Here's how the part is built. I have some questions about the finished solid (model axes, mm). Face numbers are marked on the shaded views. A direction names the side the tool comes from. Round coordinates to 2 decimals unless told otherwise and drop trailing zeros. Order: outer loops, then holes, each group sorted by start corner. A loop starts at its lowest first (then second) coordinate and runs counter-clockwise, first axis right, second up. Notation, with made-up numbers: (67, 8.5) -> (118, 8.5) arc R27 cw to (118, 27.5) -> close; hole circle Ø6 at (-19.5, 0). An arc over 180 degrees is marked (long way). Use a Markdown table: item, result. Add a question column.
(1) I want a section at C-C, the plane x = 30.5. Please give me the cut outline in (y, z), then the cut area to 3 significant figures.
(2) I'm going to push flat-ended pins straight in: P1, Ø3.5, axis at x = 8, z = -33.18, coming from the +Y side; P2, Ø1, axis at x = 62.5, z = -46.5, coming from the -Y side; P3, Ø2.5, axis at x = 26, z = 17.32, coming from the +Y side. Where does each tip first touch, or does it pass through?
(3) If I drill on probe 1 along Y at (x, z) = (73, -17); probe 2 along X at (y, z) = (8, -62); probe 3 along Z at (x, y) = (42, 6), over which ranges is the centre line in solid material (lowest first)?
(4) Thinking about a two-plate mould opening in Y: for the marked faces 1, 2 and 3, which applies, pulls with the +Y half, pulls with the -Y half, needs draft (parallel to the pull), parting line crosses it, or undercut?
(5) On a 3-axis mill with a long thin cutter (end or side, diameter ignored), from which of +Z, -Z, +X, -X, +Y, -Y can I reach the whole of each face in a straight line? I mean the marked faces 4, 5 and 6. Say none if no direction works.
(6) I want a section at D-D, the plane z = -47. Please give me the cut outline in (x, y), then the cut area to 3 significant figures.
(7) I want a section at B-B, the plane x = 40. Give the number of separate pieces and of enclosed holes in the cut face, then the cut area to 3 significant figures.
(8) I want a section at A-A, the plane z = 4. Please give me the cut outline in (x, y), then the cut area to 3 significant figures.
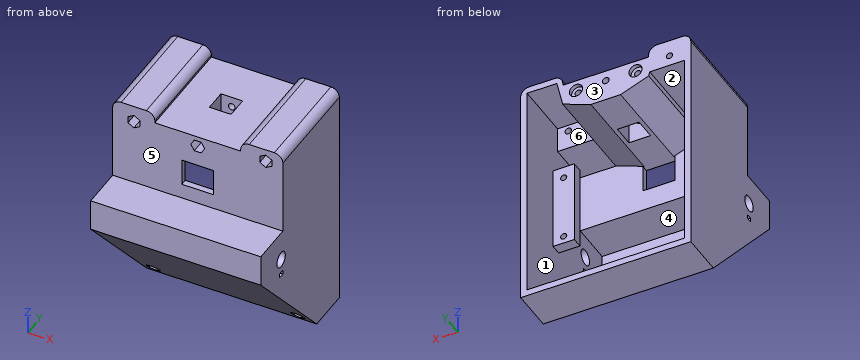
from build123d import *

# Parameters (mm, degrees)
BOSS_EXTRUDE1_DEPTH = 80
SHELL1_T            = -3
SKETCH3_W           = 46
SKETCH3_H           = 47
BOSS_EXTRUDE2_DEPTH = 17
SKETCH4_W           = 10.2
SKETCH4_H           = 10.2
CUT_EXTRUDE1_DEPTH  = 20
SKETCH6_W           = 15
SKETCH6_H           = 12.8
CUT_EXTRUDE2_DEPTH  = 3
SKETCH7_W           = 40.4
SKETCH7_H           = 50
CUT_EXTRUDE3_DEPTH  = 5
FILLET1_R           = 4
CUT_EXTRUDE7_DEPTH  = 47
SKETCH13_R          = 1.5
CUT_EXTRUDE8_DEPTH  = 25
SKETCH14_R          = 3.1
CUT_EXTRUDE9_DEPTH  = 2
SKETCH17_W          = 45
SKETCH17_H          = 5
BOSS_EXTRUDE5_DEPTH = 74
CUT_EXTRUDE10_REACH = 126.093
SKETCH18_W          = 54
SKETCH18_H          = 45
CUT_EXTRUDE11_REACH = 126.093
SKETCH19_R          = 1.45
BOSS_EXTRUDE6_DEPTH = 47
SKETCH22_R          = 1.45
CUT_EXTRUDE12_DEPTH = 135.415364765
SKETCH24_R          = 3.7
SKETCH24_W          = 2
SKETCH24_H          = 3
CUT_EXTRUDE13_DEPTH = 125.856940719
BOSS_EXTRUDE7_DEPTH = 74
SKETCH27_R          = 1.5
CUT_EXTRUDE14_DEPTH = 10
CUT_EXTRUDE15_START = -3
CUT_EXTRUDE15_DEPTH = 32
CUT_EXTRUDE16_DEPTH = 30
BOSS_EXTRUDE8_DEPTH = 20
SKETCH31_R          = 1.5
CUT_EXTRUDE17_DEPTH = 123.649786567
CUT_EXTRUDE18_DEPTH = 15
CUT_EXTRUDE19_REACH = 126.093
SKETCH33_W          = 10
SKETCH33_H          = 5
SKETCH34_R          = 1.6
CUT_EXTRUDE20_DEPTH = 135.415364765
CUT_EXTRUDE22_DEPTH = 14


with BuildPart() as part:
    # Sketch2 → Boss-Extrude1 (new body)
    with BuildSketch(Plane(origin=(0, 0, 0), x_dir=(0, 0, -1), z_dir=(1, 0, 0))):
        Polygon((-27.320490368, 20.998248687), (-27.320490368, -29.001751313), (12.679509632, -29.001751313), (12.679509632, -48.511383538), (27.679509632, -48.511383538), (82.679509632, 0.998248687), (82.679509632, 20.998248687), align=None)
    extrude(amount=BOSS_EXTRUDE1_DEPTH)

    # Shell1
    shell1_openings = [part.faces().sort_by_distance(p)[0] for p in [
        (40, 20.998248687, -27.679509632),
    ]]
    offset(amount=SHELL1_T, openings=shell1_openings, kind=Kind.INTERSECTION)

    # Sketch3 → Boss-Extrude2 (add)
    with BuildSketch(Plane(origin=(0, 0, 24.320490368), x_dir=(-1, 0, 0), z_dir=(0, 0, -1))):
        with Locations((-40, -2.501751313)):
            Rectangle(SKETCH3_W, SKETCH3_H)
    extrude(amount=BOSS_EXTRUDE2_DEPTH)

    # Sketch4 → Cut-Extrude1 (cut)
    with BuildSketch(Plane.XY.offset(27.320490368)):
        with Locations((40, -4.001751313)):
            Rectangle(SKETCH4_W, SKETCH4_H)
    extrude(amount=-CUT_EXTRUDE1_DEPTH, mode=Mode.SUBTRACT)

    # Sketch6 → Cut-Extrude2 (cut)
    with BuildSketch(Plane.XZ.offset(29.001751313)):
        with Locations((40, 0.920490368)):
            Rectangle(SKETCH6_W, SKETCH6_H)
    extrude(amount=-CUT_EXTRUDE2_DEPTH, mode=Mode.SUBTRACT)

    # Sketch7 → Cut-Extrude3 (cut)
    with BuildSketch(Plane.XY.offset(27.320490368)):
        with Locations((40, -4.001751313)):
            Rectangle(SKETCH7_W, SKETCH7_H)
    extrude(amount=-CUT_EXTRUDE3_DEPTH, mode=Mode.SUBTRACT)

    # Fillet1
    fillet1_edges = [part.edges().sort_by_distance(p)[0] for p in [
        (80, -4.001751313, 27.320490368),
        (19.8, -4.001751313, 27.320490368),
        (0, -4.001751313, 27.320490368),
        (60.2, -4.001751313, 27.320490368),
    ]]
    fillet(fillet1_edges, radius=FILLET1_R)

    # Sketch12 → Cut-Extrude7 (cut)
    with BuildSketch(Plane(origin=(0, 20.998248687, 0), x_dir=(1, 0, 0), z_dir=(0, 1, 0))):
        Polygon((33, -7.320490368), (19.8, -12.320490368), (17, -24.320490368), (17, -7.320490368), align=None)
        Polygon((47, -7.320490368), (63, -7.320490368), (63, -24.320490368), (60.2, -12.320490368), align=None)
    extrude(amount=-CUT_EXTRUDE7_DEPTH, mode=Mode.SUBTRACT)

    # Sketch13 → Cut-Extrude8 (cut)
    with BuildSketch(Plane(origin=(0, 20.998248687, 0), x_dir=(1, 0, 0), z_dir=(0, 1, 0))):
        with Locations(Location((26, -17.320490368, 0), (0, 0, 270))):
            Circle(SKETCH13_R)
        with Locations(Location((54, -17.320490368, 0), (0, 0, 270))):
            Circle(SKETCH13_R)
    extrude(amount=-CUT_EXTRUDE8_DEPTH, mode=Mode.SUBTRACT)

    # Sketch14 → Cut-Extrude9 (cut)
    with BuildSketch(Plane(origin=(0, 20.998248687, 0), x_dir=(1, 0, 0), z_dir=(0, 1, 0))):
        with Locations(Location((26, -17.320490368, 0), (0, 0, 270))):
            Circle(SKETCH14_R)
        with Locations(Location((54, -17.320490368, 0), (0, 0, 270))):
            Circle(SKETCH14_R)
    extrude(amount=-CUT_EXTRUDE9_DEPTH, mode=Mode.SUBTRACT)

    # Sketch17 → Boss-Extrude5 (add)
    with BuildSketch(Plane.ZY.offset(-77)):
        with Locations((-23.179509632, -4.501751313)):
            Rectangle(SKETCH17_W, SKETCH17_H)
    extrude(amount=BOSS_EXTRUDE5_DEPTH)

    # Sketch18 → Cut-Extrude10 (cut, up to next)
    with BuildSketch(Plane(origin=(0, -2.001751313, 0), x_dir=(1, 0, 0), z_dir=(0, 1, 0)), mode=Mode.PRIVATE) as cut_extrude10_sk1:
        with Locations((40, 23.179509632)):
            Rectangle(SKETCH18_W, SKETCH18_H)
    cut_extrude10_tool1 = extrude(cut_extrude10_sk1.sketch, amount=-CUT_EXTRUDE10_REACH, mode=Mode.PRIVATE) & part.part
    add(cut_extrude10_tool1.solids().sort_by_distance((40, -2.001751, -23.17951))[0], mode=Mode.SUBTRACT)

    # Sketch19 → Cut-Extrude11 (cut, up to next)
    with BuildSketch(Plane(origin=(0, -2.001751313, 0), x_dir=(1, 0, 0), z_dir=(0, 1, 0)), mode=Mode.PRIVATE) as cut_extrude11_sk1:
        with Locations(Location((72, 37.179509632, 0), (0, 0, 270))):
            Circle(SKETCH19_R)
    cut_extrude11_tool1 = extrude(cut_extrude11_sk1.sketch, amount=-CUT_EXTRUDE11_REACH, mode=Mode.PRIVATE) & part.part
    # Sketch19 → Cut-Extrude11 (cut, up to next)
    with BuildSketch(Plane(origin=(0, -2.001751313, 0), x_dir=(1, 0, 0), z_dir=(0, 1, 0)), mode=Mode.PRIVATE) as cut_extrude11_sk2:
        with Locations(Location((72, 6.179509632, 0), (0, 0, 270))):
            Circle(SKETCH19_R)
    cut_extrude11_tool2 = extrude(cut_extrude11_sk2.sketch, amount=-CUT_EXTRUDE11_REACH, mode=Mode.PRIVATE) & part.part
    # Sketch19 → Cut-Extrude11 (cut, up to next)
    with BuildSketch(Plane(origin=(0, -2.001751313, 0), x_dir=(1, 0, 0), z_dir=(0, 1, 0)), mode=Mode.PRIVATE) as cut_extrude11_sk3:
        with Locations(Location((8, 33.179509632, 0), (0, 0, 270))):
            Circle(SKETCH19_R)
    cut_extrude11_tool3 = extrude(cut_extrude11_sk3.sketch, amount=-CUT_EXTRUDE11_REACH, mode=Mode.PRIVATE) & part.part
    # Sketch19 → Cut-Extrude11 (cut, up to next)
    with BuildSketch(Plane(origin=(0, -2.001751313, 0), x_dir=(1, 0, 0), z_dir=(0, 1, 0)), mode=Mode.PRIVATE) as cut_extrude11_sk4:
        with Locations(Location((8, 6.179509632, 0), (0, 0, 270))):
            Circle(SKETCH19_R)
    cut_extrude11_tool4 = extrude(cut_extrude11_sk4.sketch, amount=-CUT_EXTRUDE11_REACH, mode=Mode.PRIVATE) & part.part
    add(cut_extrude11_tool1.solids().sort_by_distance((72, -2.001751, -37.17951))[0], mode=Mode.SUBTRACT)
    add(cut_extrude11_tool2.solids().sort_by_distance((72, -2.001751, -6.17951))[0], mode=Mode.SUBTRACT)
    add(cut_extrude11_tool3.solids().sort_by_distance((8, -2.001751, -33.17951))[0], mode=Mode.SUBTRACT)
    add(cut_extrude11_tool4.solids().sort_by_distance((8, -2.001751, -6.17951))[0], mode=Mode.SUBTRACT)

    # Sketch21 → Boss-Extrude6 (add)
    with BuildSketch(Plane(origin=(0, -26.001751313, 0), x_dir=(1, 0, 0), z_dir=(0, 1, 0))):
        Polygon((3, -24.320490368), (3, -14.320490368), (19.333333333, -14.320490368), (17, -24.320490368), align=None)
    extrude(amount=BOSS_EXTRUDE6_DEPTH)

    # Sketch22 → Cut-Extrude12 (cut, through all)
    with BuildSketch(Plane(origin=(0, 20.998248687, 0), x_dir=(1, 0, 0), z_dir=(0, 1, 0))):
        with Locations(Location((10, -19.320490368, 0), (0, 0, 270))):
            Circle(SKETCH22_R)
    extrude(amount=-CUT_EXTRUDE12_DEPTH, mode=Mode.SUBTRACT)

    # Sketch24 → Cut-Extrude13 (cut, through all)
    with BuildSketch(Plane(origin=(80, 0, 0), x_dir=(0, 0, -1), z_dir=(1, 0, 0))):
        with Locations((26.679509632, -30.511383538)):
            Circle(SKETCH24_R)
        with Locations((34.379509632, -30.511383538)):
            Rectangle(SKETCH24_W, SKETCH24_H)
    extrude(amount=-CUT_EXTRUDE13_DEPTH, mode=Mode.SUBTRACT)

    # Sketch26 → Boss-Extrude7 (add)
    with BuildSketch(Plane(origin=(3, 0, 0), x_dir=(0, 0, -1), z_dir=(1, 0, 0))):
        Polygon((79.679509632, 2.334161996), (63.679509632, 2.334161996), (63.679509632, -12.068640106), align=None)
    extrude(amount=BOSS_EXTRUDE7_DEPTH)

    # Sketch27 → Cut-Extrude14 (cut)
    with BuildSketch(Plane(origin=(0, 2.334161996, 0), x_dir=(1, 0, 0), z_dir=(0, 1, 0))):
        with Locations(Location((6, 76.679509632, 0), (0, 0, 270))):
            Circle(SKETCH27_R)
        with Locations(Location((74, 76.679509632, 0), (0, 0, 270))):
            Circle(SKETCH27_R)
    extrude(amount=-CUT_EXTRUDE14_DEPTH, mode=Mode.SUBTRACT)

    # Sketch28 → Cut-Extrude15 (cut)
    with BuildSketch(Plane(origin=(0, 2.334161996, 0), x_dir=(1, 0, 0), z_dir=(0, 1, 0)).offset(CUT_EXTRUDE15_START)):
        Polygon((74, 79.929509632), (71.185417438, 78.304509632), (71.185417438, 75.054509632), (74, 73.429509632), (76.814582562, 75.054509632), (76.814582562, 78.304509632), align=None)
        Polygon((6, 73.429509632), (8.814582562, 75.054509632), (8.814582562, 78.304509632), (6, 79.929509632), (3.185417438, 78.304509632), (3.185417438, 75.054509632), align=None)
    extrude(amount=-CUT_EXTRUDE15_DEPTH, mode=Mode.SUBTRACT)

    # Sketch29 → Cut-Extrude16 (cut)
    with BuildSketch(Plane.XZ.offset(29.001751313)):
        Polygon((7.185417438, 17.695490368), (10, 16.070490368), (12.814582562, 17.695490368), (12.814582562, 20.945490368), (10, 22.570490368), (7.185417438, 20.945490368), align=None)
    extrude(amount=-CUT_EXTRUDE16_DEPTH, mode=Mode.SUBTRACT)

    # Sketch30 → Boss-Extrude8 (add)
    with BuildSketch(Plane(origin=(0, -26.001751313, 0), x_dir=(1, 0, 0), z_dir=(0, 1, 0))):
        Polygon((77, -24.320490368), (63, -24.320490368), (60.2, -12.320490368), (77, -12.320490368), align=None)
    extrude(amount=BOSS_EXTRUDE8_DEPTH)

    # Sketch31 → Cut-Extrude17 (cut, through all)
    with BuildSketch(Plane(origin=(0, -6.001751313, 0), x_dir=(1, 0, 0), z_dir=(0, 1, 0))):
        with Locations(Location((72, -21.320490368, 0), (0, 0, 270))):
            Circle(SKETCH31_R)
    extrude(amount=-CUT_EXTRUDE17_DEPTH, mode=Mode.SUBTRACT)

    # Sketch32 → Cut-Extrude18 (cut)
    with BuildSketch(Plane.XZ.offset(29.001751313)):
        Polygon((72, 24.570490368), (69.185417438, 22.945490368), (69.185417438, 19.695490368), (72, 18.070490368), (74.814582562, 19.695490368), (74.814582562, 22.945490368), align=None)
    extrude(amount=-CUT_EXTRUDE18_DEPTH, mode=Mode.SUBTRACT)

    # Sketch33 → Cut-Extrude19 (cut, up to next)
    with BuildSketch(Plane(origin=(0, -2.001751313, 0), x_dir=(1, 0, 0), z_dir=(0, 1, 0)), mode=Mode.PRIVATE) as cut_extrude19_sk1:
        with Locations((72, 43.179509632)):
            Rectangle(SKETCH33_W, SKETCH33_H)
    cut_extrude19_tool1 = extrude(cut_extrude19_sk1.sketch, amount=-CUT_EXTRUDE19_REACH, mode=Mode.PRIVATE) & part.part
    add(cut_extrude19_tool1.solids().sort_by_distance((72, -2.001751, -43.17951))[0], mode=Mode.SUBTRACT)

    # Sketch34 → Cut-Extrude20 (cut, through all)
    with BuildSketch(Plane(origin=(0, 20.998248687, 0), x_dir=(1, 0, 0), z_dir=(0, 1, 0))):
        with Locations(Location((40, -17.320490368, 0), (0, 0, 270))):
            Circle(SKETCH34_R)
    extrude(amount=-CUT_EXTRUDE20_DEPTH, mode=Mode.SUBTRACT)

    # Sketch36 → Cut-Extrude22 (cut)
    with BuildSketch(Plane.XZ.offset(29.001751313)):
        Polygon((38.375, 20.13507293), (36.75, 17.320490368), (38.375, 14.505907805), (41.625, 14.505907805), (43.25, 17.320490368), (41.625, 20.13507293), align=None)
    extrude(amount=-CUT_EXTRUDE22_DEPTH, mode=Mode.SUBTRACT)


solid = part.part
Taken from the geometry:
| question | item | result |
|---|---|---|
| 1 | outline | (-48.51, -27.68) -> (1, -82.68) -> (21, -82.68) -> (21, -79.68) -> (2.33, -79.68) -> (2.33, -63.68) -> (-12.07, -63.68) -> (-45.51, -26.53) -> (-45.51, -15.68) -> (-26, -15.68) -> (-26, 8.27) -> (21, 8.27) -> (21, 22.32) -> (-29, 22.32) -> (-29, -12.68) -> (-48.51, -12.68) -> close |
| 1 | area | 1,260 mm2 |
| 2 | P1 | stops at y = -2 |
| 2 | P2 | stops at y = -32.02 |
| 2 | P3 | stops at y = -4 |
| 3 | probe 1 | y = -48.51 to -45.51, -7 to -2 |
| 3 | probe 2 | x = 0 to 3, 77 to 80 |
| 3 | probe 3 | z = -82.68 to -79.68, 7.32 to 22.32 |
| 4 | face 1 | undercut |
| 4 | face 2 | needs draft |
| 4 | face 3 | pulls with the +Y half |
| 5 | face 4 | none |
| 5 | face 5 | +Z, +X, -X, -Y |
| 5 | face 6 | +Y |
| 6 | outline | (0, -31.12) -> (80, -31.12) -> (80, 21) -> (77, 21) -> (77, -27.08) -> (3, -27.08) -> (3, 21) -> (0, 21) -> close |
| 6 | area | 611 mm2 |
| 7 | separate pieces | 5 |
| 7 | enclosed holes | 0 |
| 7 | area | 951 mm2 |
| 8 | outline | (0, -29) -> (32.5, -29) -> (32.5, -26) -> (3, -26) -> (3, 21) -> (0, 21) -> close; (47.5, -29) -> (80, -29) -> (80, 21) -> (77, 21) -> (77, -26) -> (47.5, -26) -> close |
| 8 | area | 477 mm2 |
